Solid Edge part; units mm, degrees
sketch "Sketch1" plane through (0, 0, 0) normal (0, 0, 1) x (1, 0, 0)
  line L0 (105.1974, 149.4572) -> (268.1974, 149.4572)
  line L1 (268.1974, 149.4572) -> (268.1974, 19.4572)
  line L2 (268.1974, 19.4572) -> (105.1974, 19.4572)
  line L3 (105.1974, 19.4572) -> (105.1974, 149.4572)
  dimension "D1" = 105.1974
  dimension "D2" = 268.1974
extrude "Protrusion1" add sketch "Sketch1" along normal blind 27
sketch "Sketch2" plane through (170.1974, 84.4572, 27) normal (0, 0, 1) x (1, 0, 0)
  line L0 (-62, 62) -> (-62, -62)
  line L1 (-62, -62) -> (95, -62)
  line L2 (95, -62) -> (95, 62.14)
  line L3 (-62, 62) -> (95, 62.14)
  dimension "D1" = 62
  dimension "D2" = 95
extrude "ExtrudedCutout_1" cut sketch "Sketch2" against normal blind 23
sketch "Sketch3" plane through (170.1974, 84.5136, 4) normal (0, 0, 1) x (1, 0, 0)
  circle A0 centre (-57, -0.0564) radius 2
  circle A1 centre (-48, -0.0564) radius 2
extrude "Cutout1" cut sketch "Sketch3" against normal through all
extrude "Cutout2" [suppressed]
extrude "ExtrudedCutout_4" [suppressed]
sketch "Sketch4" plane through (105.1974, 84.4572, 12) normal (-1, 0, 0) x (0, -1, 0)
  line L0 (19.6475, 9.8237) -> (19.6475, -8)
  line L1 (19.6475, -8) -> (36.7322, -8)
  line L2 (36.7322, -8) -> (36.7322, 9.8237)
  line L3 (36.7322, 9.8237) -> (19.6475, 9.8237)
extrude "Cutout3" cut sketch "Sketch4" against normal up to next
extrude "Cutout4" [suppressed]
extrude "Cutout5" [suppressed]
Check sheet for the modelled part. Datum: model origin and axes. Units: mm. A direction names the side the tool comes from. Coordinates: 2 decimals unless noted, no trailing zeros. Order: outer loops, then holes, each group sorted by start corner. A loop starts at its lowest first (then second) coordinate and runs counter-clockwise, first axis right, second up. Notation, with made-up numbers: M 87,65 L 94,65 A9 cw 94,81 Z; hole C 6.25,47.5 d10. An arc over 180 degrees is marked long. One line per question, with ' | ' between items. Start each with the question number.
Item 1: Sectioned sample at D-D on x = 237. Record the cut outline in (y, z), and give its area (3 significant figures).
Item 2: Gauge pin test, flat end, axial feed: P1, Ø5, axis at x = 122.2, y = 84.46, coming from the +Z side. Record the tip position at first contact, or that the pin passes through.
Item 3: Mould release check, pull along X, two halves, no side actions. Record for faces 1 (the flat face through (105.197, 84, 13)), 2 (the flat face through (268.197, 85, 13)), 3 (the flat face through (184, 85, 4)), 4 (the flat face through (266, 85, 27)): pulls with the +X half, pulls with the -X half, needs draft (parallel to the pull), parting line crosses it, or undercut.
Item 4: Access from +Z, -Z, +X, -X, +Y, -Y to the whole of each face (thin tool, end or side, straight path). Record for faces 5 (the flat face through (108.197, 85, 16)), 6 (the flat face through (186, 149.457, 13)).
Item 5: Sectioned sample at C-C on z = 14.25. Record the cut outline in (x, y) (3 decimals).
Item 6: Sectioned sample at B-B on y = 101. Record the cut outline in (x, z).
Item 7: Sectioned sample at A-A on y = 56. Record the cut outline in (x, z).
Item 8: Material ranges on line 1 (X direction, y = 126, z = 17); line 2 (Y direction, x = 232.5, z = 11); line 3 (Y direction, x = 138, z = 22.5), recorded low to high.
Answer below:
1) outline: M 19.46,0 L 149.46,0 L 149.46,27 L 146.57,27 L 146.57,4 L 22.46,4 L 22.46,27 L 19.46,27 Z | area: 655 mm^2
2) P1: stops at z = 4
3) face 1: pulls with the -X half | face 2: pulls with the +X half | face 3: undercut | face 4: needs draft
4) face 5: +Z | face 6: +Z, -Z, +X, -X, +Y
5) outline: M 105.197,19.457 L 268.197,19.457 L 268.197,149.457 L 105.197,149.457 L 105.197,64.81 L 108.197,64.81 L 108.197,146.457 L 265.197,146.597 L 265.197,22.457 L 108.197,22.457 L 108.197,47.725 L 105.197,47.725 Z
6) outline: M 105.2,0 L 268.2,0 L 268.2,27 L 265.2,27 L 265.2,4 L 108.2,4 L 108.2,27 L 105.2,27 Z
7) outline: M 105.2,0 L 268.2,0 L 268.2,27 L 265.2,27 L 265.2,4 L 105.2,4 Z; M 105.2,21.82 L 108.2,21.82 L 108.2,27 L 105.2,27 Z
8) line 1: x = 105.2 to 108.2, 265.2 to 268.2 | line 2: y = 19.46 to 22.46, 146.57 to 149.46 | line 3: y = 19.46 to 22.46, 146.48 to 149.46
